The listing builds one solid part. Answer for the finished solid, in the listing's coordinates (mm). Face numbers are marked on the shaded views. A direction names the side the tool comes from. Coordinates: 2 decimals unless noted, no trailing zeros. Loops run counter-clockwise (first coordinate to the right, second up) from the corner with the lowest first, then second, coordinate; pieces in that order, holes last. Notation, with made-up numbers: M 36,89 L 88,89 A8 cw 88,104 Z; hole C 82,71.25 d5. An arc over 180 degrees is marked long. Answer as a JSON object with one key per item and string values. Group by question number.
1. Given pin 1 (3.5 mm diameter, centred on x = -22.5, z = 6.5, fed in from +Y); pin 2 (1.5 mm diameter, centred on x = 0, z = -1.5, fed in from +Y), each flat-ended and moving along its own axis, determine where each tip first touches the part or whether it passes through.
2. A cutting plane is placed at A-A on x = 15. Give the vertices of the cut face in (y, z).
3. Straight lines are drawn through the part: L1, parallel to X at y = 0.75, z = 0; L2, parallel to X at y = 8.5, z = 2; L3, parallel to X at y = 14, z = -1.5. For each, find the intervals that lie inside material, in ascending order.
4. A cutting plane is placed at C-C on z = 6.75. Give the vertices of the cut face in (x, y), and give its area (3 significant figures).
5. A cutting plane is placed at B-B on y = 12. Give the vertices of the cut face in (x, z).
6. A cutting plane is placed at D-D on x = -33. Give the vertices of the cut face in (y, z).
7. Determine the mould class of the marked faces 1, 2 and 3 for opening direction X: released by +X, released by -X, zero draft, split by the parting line, or undercut.
8. For the marked faces 4 and 5, determine the directions among +Z, -Z, +X, -X, +Y, -Y from which every point of the face is accessible in a straight line to the end or side of a thin tool.
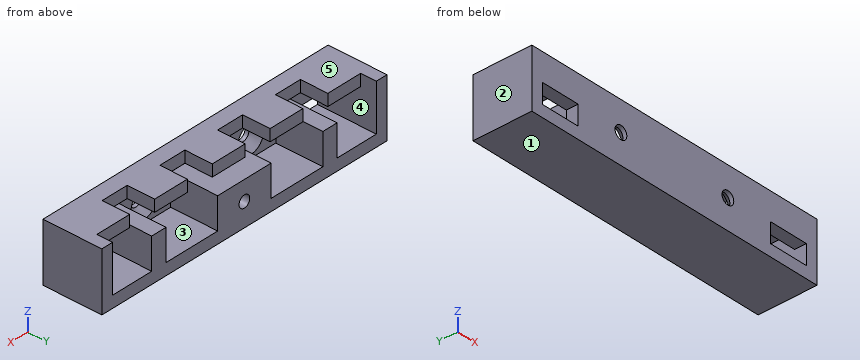
from build123d import *

# Parameters (mm, degrees)
SKETCH1_W      = 80
SKETCH1_H      = 15
SKETCH1_R      = 1.65
SKETCH1_W_2    = 10
SKETCH1_H_2    = 5
EXTRUDE1_DEPTH = 3
SKETCH2_W      = 3
SKETCH2_H      = 3
SKETCH2_H_2    = 9
SKETCH2_W_2    = 74
EXTRUDE2_DEPTH = 12
SKETCH3_W      = 7
SKETCH3_H      = 7
EXTRUDE3_DEPTH = 5
CHAMFER2_SIZE  = 2
CHAMFER3_SIZE  = 2
SKETCH4_W      = 15
SKETCH4_H      = 8
SKETCH4_W_2    = 4
EXTRUDE4_DEPTH = 12
SKETCH5_R      = 1.5
EXTRUDE5_DEPTH = 5


with BuildPart() as part:
    # Sketch1 → Extrude1 (new body)
    with BuildSketch(Plane(origin=(0, 0, 0), x_dir=(1, 0, 0), z_dir=(0, 1, 0))):
        Rectangle(SKETCH1_W, SKETCH1_H)
        with Locations((-15, 0)):
            Circle(SKETCH1_R, mode=Mode.SUBTRACT)
        with Locations((15, 0)):
            Circle(SKETCH1_R, mode=Mode.SUBTRACT)
        with Locations((-32, 2)):
            Rectangle(SKETCH1_W_2, SKETCH1_H_2, mode=Mode.SUBTRACT)
        with Locations((32, 2)):
            Rectangle(SKETCH1_W_2, SKETCH1_H_2, mode=Mode.SUBTRACT)
    extrude(amount=EXTRUDE1_DEPTH)

    # Sketch2 → Extrude2 (add)
    with BuildSketch(Plane(origin=(0, 3, 0), x_dir=(1, 0, 0), z_dir=(0, 1, 0))):
        with Locations((-38.5, 6)):
            Rectangle(SKETCH2_W, SKETCH2_H)
        with Locations((-38.5, 0)):
            Rectangle(SKETCH2_W, SKETCH2_H_2)
        with Locations((0, 6)):
            Rectangle(SKETCH2_W_2, SKETCH2_H)
        with Locations((-38.5, -6)):
            Rectangle(SKETCH2_W, SKETCH2_H)
        with Locations((0, -6)):
            Rectangle(SKETCH2_W_2, SKETCH2_H)
        with Locations((38.5, 6)):
            Rectangle(SKETCH2_W, SKETCH2_H)
        with Locations((38.5, 0)):
            Rectangle(SKETCH2_W, SKETCH2_H_2)
        with Locations((38.5, -6)):
            Rectangle(SKETCH2_W, SKETCH2_H)
    extrude(amount=EXTRUDE2_DEPTH)

    # Sketch3 → Extrude3 (cut)
    with BuildSketch(Plane.XY.offset(7.5)):
        Polygon((-20.8, 11), (-11.6, 11), (-4.6, 11), (4.6, 11), (11.6, 11), (20.8, 11), (27.8, 11), (37, 11), (37, 15), (-37, 15), (-37, 11), (-27.8, 11), align=None)
        with Locations((-24.3, 7.5)):
            Rectangle(SKETCH3_W, SKETCH3_H)
        with Locations((-8.1, 7.5)):
            Rectangle(SKETCH3_W, SKETCH3_H)
        with Locations((8.1, 7.5)):
            Rectangle(SKETCH3_W, SKETCH3_H)
        with Locations((24.3, 7.5)):
            Rectangle(SKETCH3_W, SKETCH3_H)
    extrude(amount=-EXTRUDE3_DEPTH, mode=Mode.SUBTRACT)

    # Chamfer2
    chamfer2_edges = [part.edges().sort_by_distance(p)[0] for p in [
        (13.35, 3, 0),
    ]]
    chamfer(chamfer2_edges, length=CHAMFER2_SIZE)

    # Chamfer3
    chamfer3_edges = [part.edges().sort_by_distance(p)[0] for p in [
        (-16.65, 3, 0),
    ]]
    chamfer(chamfer3_edges, length=CHAMFER3_SIZE)

    # Sketch4 → Extrude4 (add)
    with BuildSketch(Plane(origin=(0, 3, 0), x_dir=(1, 0, 0), z_dir=(0, 1, 0))):
        with Locations((0, 0.5)):
            Rectangle(SKETCH4_W, SKETCH4_H)
        with Locations((-24, 0.5)):
            Rectangle(SKETCH4_W_2, SKETCH4_H)
        with Locations((24, 0.5)):
            Rectangle(SKETCH4_W_2, SKETCH4_H)
    extrude(amount=EXTRUDE4_DEPTH)

    # Sketch5 → Extrude5 (cut)
    with BuildSketch(Plane(origin=(0, 15, 0), x_dir=(1, 0, 0), z_dir=(0, 1, 0))):
        with Locations((0, 1.5)):
            Circle(SKETCH5_R)
    extrude(amount=-EXTRUDE5_DEPTH, mode=Mode.SUBTRACT)


solid = part.part
From the geometry:
{
 "1": {"pin 1": "stops at y = 11", "pin 2": "stops at y = 10"},
 "2": {"outline": "M 0,-7.5 L 15,-7.5 L 15,-4.5 L 3,-4.5 L 3,-3.65 L 1,-1.65 L 0,-1.65 Z; M 0,1.65 L 1,1.65 L 3,3.65 L 3,4.5 L 11,4.5 L 11,7.5 L 0,7.5 Z"},
 "3": {"L1": "x = -40 to -37, -27 to -16.65, -13.35 to 13.35, 16.65 to 27, 37 to 40", "L2": "x = -40 to -37, -26 to -22, -7.5 to 7.5, 22 to 26, 37 to 40", "L3": "x = -40 to -37, -26 to -22, -7.5 to -1.5, 1.5 to 7.5, 22 to 26, 37 to 40"},
 "4": {"outline": "M -40,0 L 40,0 L 40,15 L 37,15 L 37,11 L 27.8,11 L 27.8,4 L 20.8,4 L 20.8,11 L 11.6,11 L 11.6,4 L 4.6,4 L 4.6,11 L -4.6,11 L -4.6,4 L -11.6,4 L -11.6,11 L -20.8,11 L -20.8,4 L -27.8,4 L -27.8,11 L -37,11 L -37,15 L -40,15 Z", "area": "708 mm²"},
 "5": {"outline": "M -40,-7.5 L 40,-7.5 L 40,7.5 L 37,7.5 L 37,-4.5 L 26,-4.5 L 26,3.5 L 22,3.5 L 22,-4.5 L 7.5,-4.5 L 7.5,3.5 L -7.5,3.5 L -7.5,-4.5 L -22,-4.5 L -22,3.5 L -26,3.5 L -26,-4.5 L -37,-4.5 L -37,7.5 L -40,7.5 Z; hole C 0,-1.5 d3"},
 "6": {"outline": "M 0,-7.5 L 15,-7.5 L 15,-4.5 L 0,-4.5 Z; M 0,0.5 L 3,0.5 L 3,4.5 L 11,4.5 L 11,7.5 L 0,7.5 Z"},
 "7": {"face 1": "zero draft", "face 2": "released by -X", "face 3": "undercut"},
 "8": {"face 4": "+Y", "face 5": "+Z, +X, -X, +Y, -Y"}
}
